For this review, take the finished solid that the model builds, in its own axes (mm). A direction names the side the tool comes from. Coordinates: 2 decimals unless noted, no trailing zeros. Loops run counter-clockwise (first coordinate to the right, second up) from the corner with the lowest first, then second, coordinate; pieces in that order, holes last. Notation, with made-up numbers: (24, 17) -> (65, 17) arc R6 cw to (65, 28) -> close; hole circle Ø11 at (69, 75.5). An arc over 180 degrees is marked (long way). Use a Markdown table: item, result.
from build123d import *

# Parameters (mm, degrees)
SKETCH2_W           = 42.3
SKETCH2_H           = 42.3
SKETCH2_R           = 1.5
SKETCH2_R_2         = 12
BOSS_EXTRUDE1_DEPTH = 5
SKETCH5_W           = 5
SKETCH5_H           = 42.3
BOSS_EXTRUDE3_DEPTH = 5
SKETCH3_W           = 20
SKETCH3_H           = 70
SKETCH3_R           = 2.75
BOSS_EXTRUDE2_DEPTH = 5
FILLET1_R           = 4


with BuildPart() as part:
    # Sketch2 → Boss-Extrude1 (new body)
    with BuildSketch(Plane(origin=(0, 0, 0), x_dir=(0, 0, -1), z_dir=(1, 0, 0))):
        Rectangle(SKETCH2_W, SKETCH2_H)
        with Locations((-15.5, 15.5)):
            Circle(SKETCH2_R, mode=Mode.SUBTRACT)
        with Locations((15.5, 15.5)):
            Circle(SKETCH2_R, mode=Mode.SUBTRACT)
        with Locations((15.5, -15.5)):
            Circle(SKETCH2_R, mode=Mode.SUBTRACT)
        with Locations((-15.5, -15.5)):
            Circle(SKETCH2_R, mode=Mode.SUBTRACT)
        Circle(SKETCH2_R_2, mode=Mode.SUBTRACT)
    extrude(amount=BOSS_EXTRUDE1_DEPTH)

    # Sketch5 → Boss-Extrude3 (add)
    with BuildSketch(Plane.XY.offset(21.15)):
        with Locations((2.5, 0)):
            Rectangle(SKETCH5_W, SKETCH5_H)
    extrude(amount=BOSS_EXTRUDE3_DEPTH)

    # Sketch3 → Boss-Extrude2 (add)
    with BuildSketch(Plane.XY.offset(26.15)):
        with Locations((10, 0)):
            Rectangle(SKETCH3_W, SKETCH3_H)
        with Locations((10, 28)):
            Circle(SKETCH3_R, mode=Mode.SUBTRACT)
        with Locations((10, -28)):
            Circle(SKETCH3_R, mode=Mode.SUBTRACT)
    extrude(amount=BOSS_EXTRUDE2_DEPTH)

    # Fillet1
    fillet1_edges = [part.edges().sort_by_distance(p)[0] for p in [
        (2.5, -21.15, 26.15),
        (2.5, 21.15, 26.15),
    ]]
    fillet(fillet1_edges, radius=FILLET1_R)


solid = part.part
(1) Take a section at A-A on y = -28. Write out the cut boundary in (x, z).
Found:
| item | result |
|---|---|
| outline | (0, 26.15) -> (7.25, 26.15) -> (7.25, 31.15) -> (0, 31.15) -> close; (12.75, 26.15) -> (20, 26.15) -> (20, 31.15) -> (12.75, 31.15) -> close |
(2) For faces 4 (the face through (10, -35, 29)), 5 (the face through (5, 0, 13)), 6 (the face through (2, 21.15, 0)), list the 3-axis set-ups (+Z, -Z, +X, -X, +Y, -Y) from which the entire face can be reached by the end or side of a thin tool; tool diameter is ignored.
Found:
| item | result |
|---|---|
| face 4 | +Z, -Z, +X, -X, -Y |
| face 5 | -Z, +X, +Y, -Y |
| face 6 | -Z, +X, -X, +Y |
(3) For pin 1 Ø14 at (y, z) = (-7, 5) entering from +X; pin 2 Ø19 at (y, z) = (0, 0) entering from -X (3 decimals); pin 3 Ø1 at (x, y) = (4, -25.5) entering from -Z; pin 4 Ø5 at (y, z) = (-15.5, 15.5) entering from -X, all flat-tipped, find the tip position at first contact; note any pin that passes through.
Found:
| item | result |
|---|---|
| pin 1 | stops at x = 5 |
| pin 2 | passes through |
| pin 3 | stops at z = 26.15 |
| pin 4 | stops at x = 0 |
(4) Take a section at B-B on x = 10. Write out the cut boundary in (y, z), plus the area to 3 significant figures.
Found:
| item | result |
|---|---|
| outline | (-35, 26.15) -> (-30.75, 26.15) -> (-30.75, 31.15) -> (-35, 31.15) -> close; (-25.25, 26.15) -> (25.25, 26.15) -> (25.25, 31.15) -> (-25.25, 31.15) -> close; (30.75, 26.15) -> (35, 26.15) -> (35, 31.15) -> (30.75, 31.15) -> close |
| area | 295 mm^2 |
(5) Take a section at D-D on z = 4.5. Write out the cut boundary in (x, y).
Found:
| item | result |
|---|---|
| outline | (0, -21.15) -> (5, -21.15) -> (5, -11.12) -> (0, -11.12) -> close; (0, 11.12) -> (5, 11.12) -> (5, 21.15) -> (0, 21.15) -> close |
(6) Take a section at C-C on z = 15.5. Write out the cut boundary in (x, y).
Found:
| item | result |
|---|---|
| outline | (0, -21.15) -> (5, -21.15) -> (5, -17) -> (0, -17) -> close; (0, -14) -> (5, -14) -> (5, 14) -> (0, 14) -> close; (0, 17) -> (5, 17) -> (5, 21.15) -> (0, 21.15) -> close |
(7) Mouldability with a two-part tool opening along Z and no side actions: class faces 1 (the face through (2, -21.15, 0)), 2 (the face through (2.46, -15.43, 17)), 3 (the face through (2, 0, -21.15)) as pulls with the +Z half, pulls with the -Z half, needs draft (parallel to the pull), parting line crosses it, or undercut.
Found:
| item | result |
|---|---|
| face 1 | needs draft |
| face 2 | undercut |
| face 3 | pulls with the -Z half |
(8) For line 1 along Y through (x, z) = (3.1, -15.5); line 2 along Y through (x, z) = (10, 29.85); line 3 along Y through (x, z) = (3, 0), list the stretches that pass through material, from the lowest coordinate up.
Found:
| item | result |
|---|---|
| line 1 | y = -21.15 to -17, -14 to 14, 17 to 21.15 |
| line 2 | y = -35 to -30.75, -25.25 to 25.25, 30.75 to 35 |
| line 3 | y = -21.15 to -12, 12 to 21.15 |
